Geometry: see drawing. Coordinates: mm, zero at the bounding-box minimum. A direction names the side the tool comes from. Coordinates: 2 decimals unless noted, no trailing zeros. Loops run counter-clockwise (first coordinate to the right, second up) from the corner with the lowest first, then second, coordinate; pieces in that order, holes last. Notation, with made-up numbers: (59.5, -3) -> (101.5, -3) arc R22 ccw to (101.5, 15) -> close; hole circle Ø7 at (87.5, -5). An arc over 180 degrees is marked (long way). Put each result on its own line as item: value. Start each with the question number.
1) Cut plane B-B (x = 2.75). Return the cut outline in (y, z), plus the area to 3 significant figures.
2) Cut plane D-D (x = 5.5). Return the cut outline in (y, z).
3) Cut plane C-C (z = 1.6). Return the cut outline in (x, y), plus the area to 3 significant figures.
4) Contact query for flat-ended pins moving along their axis: P1, Ø3, axis at x = 7, y = 2, coming from the -Z side; P2, Ø1, axis at y = 2.5, z = 2.5, coming from the +X side; P3, Ø1.2, axis at x = 4.5, y = 2.5, coming from the +Z side. Output: stop coordinate, or through.
5) Pull-direction query (X, two-part tool) for the marked faces 1, 2, 3 and 4; classes: pulls with the +X half, pulls with the -X half, needs draft (parallel to the pull), parting line crosses it, or undercut.
6) Cut plane A-A (y = 6). Return the cut outline in (x, z), plus the area to 3 significant figures.
7) Set-up query: the marked faces 5, 6, 7 and 8. Return all of +Z, -Z, +X, -X, +Y, -Y with unobstructed straight access to the full face (end or side cutting, diameter ignored); none if empty.
8) Material intervals for L1, parallel to X at y = 6, z = 2.05; L2, parallel to Y at x = 3.75, z = 2.3; L3, parallel to Z at x = 9, y = 2.5, sorted ascending.
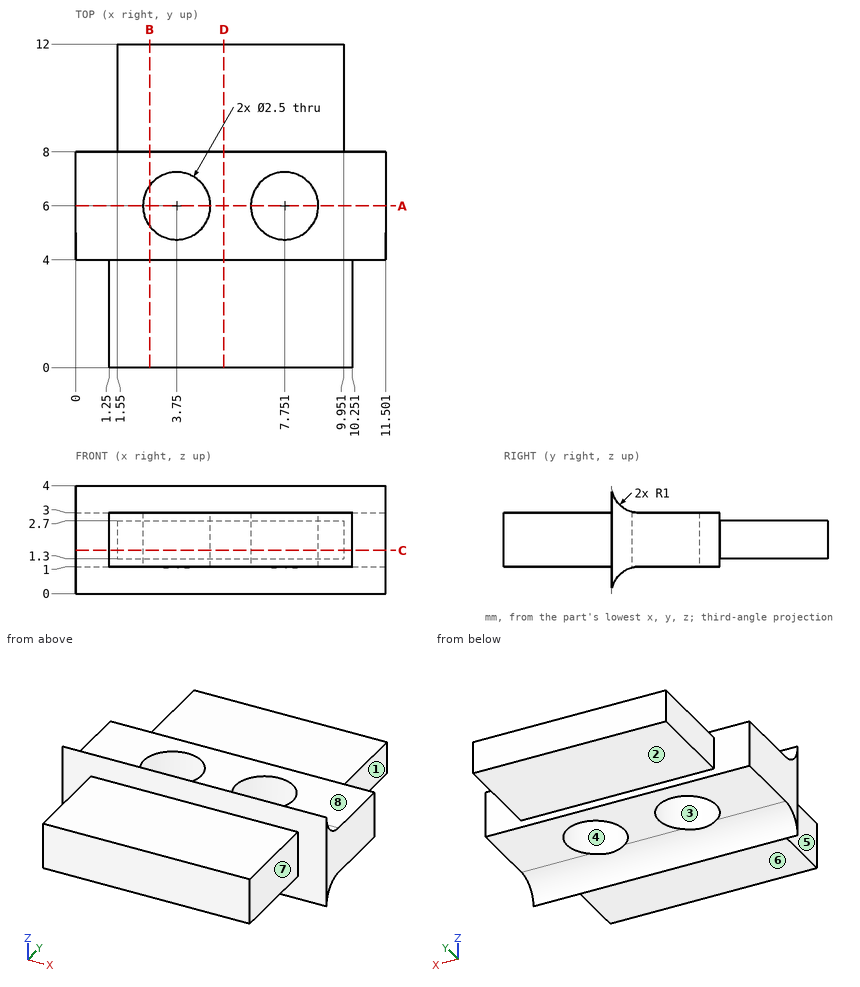
Results found:
1. outline: (0, 1) -> (4, 1) -> (4, 0) arc R1 cw to (5, 1) -> (5.25, 1) -> (5.25, 3) -> (5, 3) arc R1 cw to (4, 4) -> (4, 3) -> (0, 3) -> close; (6.75, 1) -> (8, 1) -> (8, 1.3) -> (12, 1.3) -> (12, 2.7) -> (8, 2.7) -> (8, 3) -> (6.75, 3) -> close
1. area: 19.0 mm2
2. outline: (0, 1) -> (4, 1) -> (4, 0) arc R1 cw to (5, 1) -> (8, 1) -> (8, 1.3) -> (12, 1.3) -> (12, 2.7) -> (8, 2.7) -> (8, 3) -> (5, 3) arc R1 cw to (4, 4) -> (4, 3) -> (0, 3) -> close
3. outline: (0, 4) -> (1.25, 4) -> (1.25, 0) -> (10.25, 0) -> (10.25, 4) -> (11.5, 4) -> (11.5, 8) -> (9.95, 8) -> (9.95, 12) -> (1.55, 12) -> (1.55, 8) -> (0, 8) -> close; hole circle Ø2.5 at (3.75, 6); hole circle Ø2.5 at (7.75, 6)
3. area: 106 mm2
4. P1: stops at z = 1
4. P2: stops at x = 10.25
4. P3: stops at z = 3
5. face 1: pulls with the +X half
5. face 2: needs draft
5. face 3: undercut
5. face 4: undercut
6. outline: (0, 1) -> (2.5, 1) -> (2.5, 3) -> (0, 3) -> close; (5, 1) -> (6.5, 1) -> (6.5, 3) -> (5, 3) -> close; (9, 1) -> (11.5, 1) -> (11.5, 3) -> (9, 3) -> close
6. area: 13.0 mm2
7. face 5: +Z, -Z, -X, -Y
7. face 6: -Z, +X, -X, -Y
7. face 7: +Z, -Z, +X, -Y
7. face 8: +Z, +X, -X, +Y
8. L1: x = 0 to 2.5, 5 to 6.5, 9 to 11.5
8. L2: y = 0 to 4.75, 7.25 to 12
8. L3: z = 1 to 3
